Design review of the part shown in the three views and the two pictorial views. Dimensions are in mm from the part's minimum x, y and z. A direction names the side the tool comes from. Round coordinates to 2 decimals unless told otherwise and drop trailing zeros. Loops run counter-clockwise (first coordinate to the right, second up) from the corner with the lowest first, then second, coordinate; pieces in that order, holes last. Notation, with made-up numbers: (-22.5, 32.5) -> (11.5, 32.5) arc R10 cw to (11.5, 39.5) -> close; hole circle Ø10 at (67.5, 51). An arc over 180 degrees is marked (long way). Write each question's results on one line, items separated by ' | '. Start each with the question number.
Item 1: Clearance check with flat-ended pins moving along their axes: pin 1 Ø1.5 at (x, z) = (8.5, 14.5) entering from +Y; pin 2 Ø6 at (x, z) = (11, 10) entering from -Y; pin 3 Ø1.5 at (x, z) = (5.5, 6) entering from +Y. State where each tip first meets the part, or that it passes through.
Item 2: We need section D-D (z = 1.75). Give the boundary of the cut face in (x, y), and give its area (3 significant figures).
Item 3: We need section A-A (x = 9.5). Give the boundary of the cut face in (y, z).
Item 4: For L1, parallel to Z at x = 6.75, y = 2.25; L2, parallel to Y at x = 9.25, z = 9.5; L3, parallel to Z at x = 16.75, y = 13.75, list the stretches that pass through material, from the lowest coordinate up. Write a range as from..to.
Item 5: Tool access review of the marked faces 1, 2 and 3: name each direction out of +Z, -Z, +X, -X, +Y, -Y from which nothing blocks a thin tool from reaching the whole face with its end or side.
Item 6: We need section C-C (z = 5.5). Give the boundary of the cut face in (x, y).
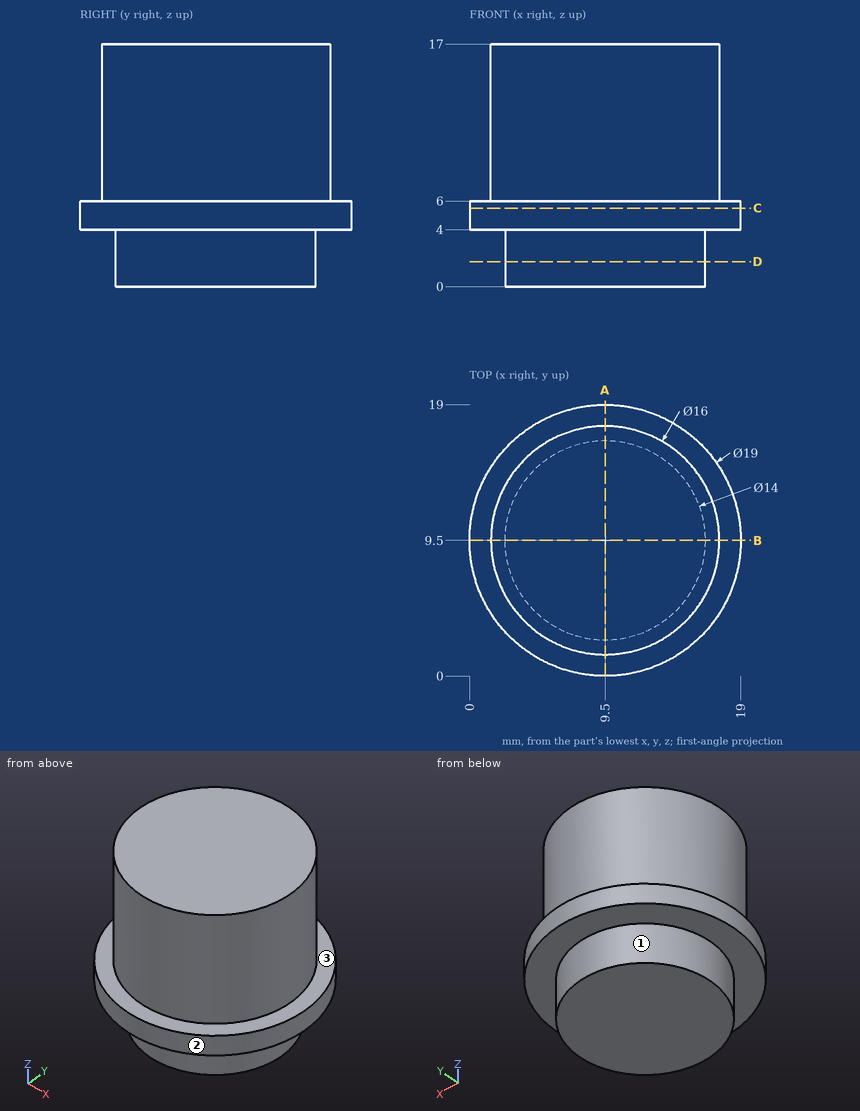
Here are the results:
1) pin 1: stops at y = 17.5 | pin 2: stops at y = 1.5 | pin 3: stops at y = 18.43
2) outline: circle Ø14 at (9.5, 9.5) | area: 154 mm2
3) outline: (0, 4) -> (2.5, 4) -> (2.5, 0) -> (16.5, 0) -> (16.5, 4) -> (19, 4) -> (19, 6) -> (17.5, 6) -> (17.5, 17) -> (1.5, 17) -> (1.5, 6) -> (0, 6) -> close
4) L1: z = 4..17 | L2: y = 1.5..17.5 | L3: z = 4..6
5) face 1: -Z | face 2: +Z, -Z | face 3: +Z
6) outline: circle Ø19 at (9.5, 9.5)
